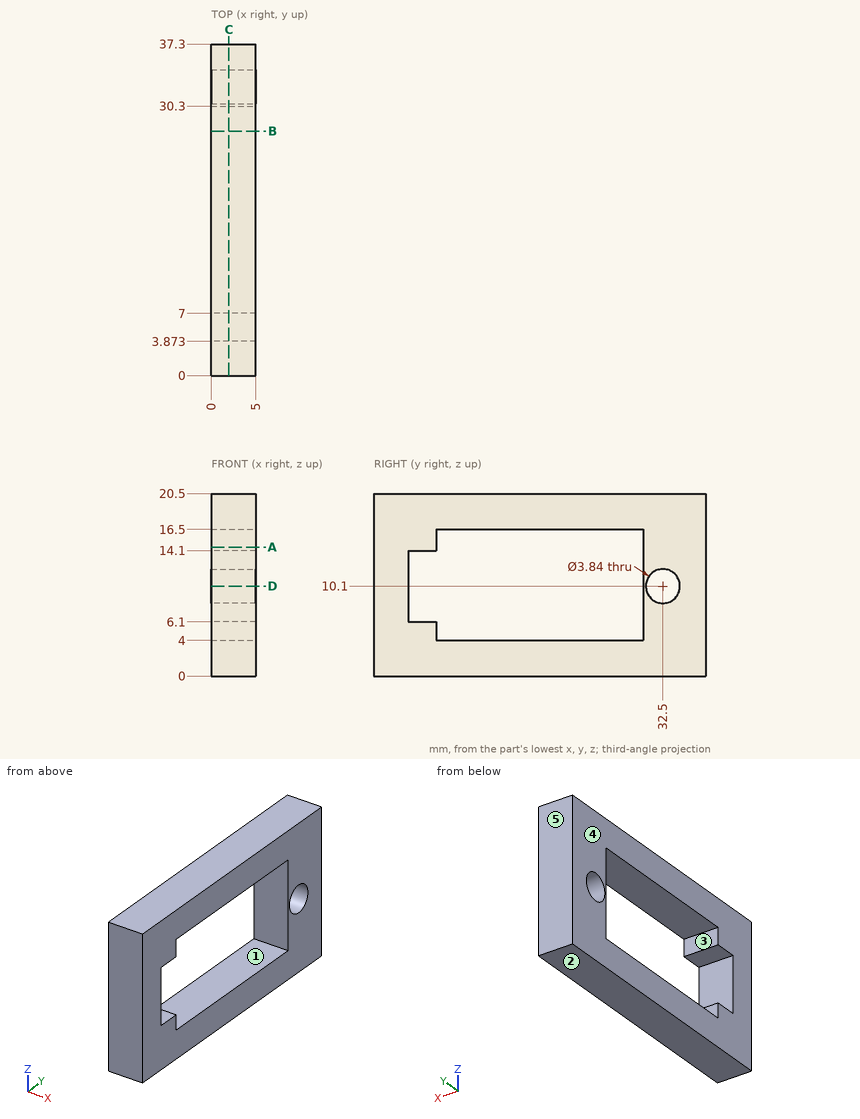
Source: three-view drawing plus pictorial views. Frame: mm from the lowest corner of the part. A direction names the side the tool comes from. Give positions to 0.01 mm unless a question says otherwise; leave off trailing zeros. Order: outer loops, then holes, each group sorted by start corner. A loop starts at its lowest first (then second) coordinate and runs counter-clockwise, first axis right, second up. Notation, with made-up numbers: M 55,31.5 L 114,31.5 A25 ccw 114,45.5 Z; hole C 33.5,43.25 d10. An arc over 180 degrees is marked long. Return JSON: item names as keys, results as strings.
Item 1: Cut plane B-B (y = 27.5). Return loops of the section in (x, z).
Solutions:
{"outline": "M 0,0 L 5,0 L 5,4 L 0,4 Z; M 0,16.5 L 5,16.5 L 5,20.5 L 0,20.5 Z"}
Item 2: Access query for the marked faces 1 and 2. Directions: +Z, -Z, +X, -X, +Y, -Y. A direction counts if a zero-diameter tool reaches every point of the face in a straight line with its end or side. Return the directions, or none.
Solutions:
{"face 1": "+X, -X", "face 2": "-Z, +X, -X, +Y, -Y"}
Item 3: Ray query, probe 1 along Z at (x, y) = (1.55, 16); probe 2 along Z at (x, y) = (1.1, 4); probe 3 along Y at (x, z) = (2.5, 10.1). Return the intervals inside material, ascending.
Solutions:
{"probe 1": "0 to 4, 16.5 to 20.5", "probe 2": "0 to 6.1, 14.1 to 20.5", "probe 3": "0 to 3.87, 30.3 to 30.58, 34.42 to 37.3"}
Item 4: Cut plane A-A (z = 14.5). Return loops of the section in (x, y), then the cut area to 3 significant figures.
Solutions:
{"outline": "M 0,0 L 5,0 L 5,7 L 0,7 Z; M 0,30.3 L 5,30.3 L 5,37.3 L 0,37.3 Z", "area": "70.0 mm^2"}
Item 5: Cut plane C-C (x = 1.95). Return loops of the section in (y, z), then the cut area to 3 significant figures.
Solutions:
{"outline": "M 0,0 L 37.3,0 L 37.3,20.5 L 0,20.5 Z; hole M 3.87,6.1 L 7,6.1 L 7,4 L 30.3,4 L 30.3,16.5 L 7,16.5 L 7,14.1 L 3.87,14.1 Z; hole C 32.5,10.1 d3.84", "area": "437 mm^2"}
Item 6: Cut plane D-D (z = 10.1). Return loops of the section in (x, y).
Solutions:
{"outline": "M 0,0 L 5,0 L 5,3.87 L 0,3.87 Z; M 0,30.3 L 5,30.3 L 5,30.58 L 0,30.58 Z; M 0,34.42 L 5,34.42 L 5,37.3 L 0,37.3 Z"}
Item 7: Pull-direction query (Y, two-part tool) for the marked faces 3, 4 and 5; classes: +Y half, -Y half, draft (parallel to the pull), parting line (faces both ways), or undercut.
Solutions:
{"face 3": "undercut", "face 4": "draft", "face 5": "+Y half"}
Item 8: First-contact query: P1, Ø3, axis at y = 32.5, z = 10.1, coming from the +X side. Flat tip, straight axial feed; report the tip coordinate or a pass-through.
Solutions:
{"P1": "through"}
